Autodesk Inventor part; units mm, degrees
ref_plane "YZ Plane" through (0, 0, 0) normal (1, 0, 0) x (0, 1, 0)
ref_plane "XZ Plane" through (0, 0, 0) normal (0, 1, 0) x (-1, 0, 0)
ref_plane "XY Plane" through (0, 0, 0) normal (0, 0, 1) x (1, 0, 0)
sketch "Sketch1" plane through (0, 0, 0) normal (0, 1, 0) x (-1, 0, 0)
  line L0 (0, 0) -> (-177.8, 0)
  line L1 (-177.8, 0) -> (-177.8, 254)
  line L2 (-177.8, 254) -> (0, 254)
  line L3 (0, 254) -> (0, 0)
  dimension "d0" = 177.8
  dimension "d1" = 254
extrude "Extrusion1" add sketch "Sketch1" along normal blind 127
shell "Shell1" thickness 3.81 removed faces 1 at (118.5333, 127, 169.3333)
sketch "Sketch2" plane through (0, 0, 254) normal (0, 0, 1) x (1, 0, 0)
  line L0 (0, 0) -> (177.8, 0)
  line L1 (177.8, 0) -> (177.8, 127)
  line L2 (0, 127) -> (177.8, 127)
  line L3 (0, 0) -> (0, 127)
extrude "Extrusion2" cut sketch "Sketch2" against normal up to surface (3.81 mm away)
sketch "Sketch3" plane through (0, 0, 0) normal (0, -1, 0) x (1, 0, 0)
  line L0 (177.8, 250.19) -> (0, 250.19)
  line L1 (0, 0) -> (0, 250.19)
  line L2 (177.8, 0) -> (0, 0)
  line L3 (177.8, 250.19) -> (177.8, 0)
  line L4 (177.8, 250.19) -> (0, 250.19)
  line L5 (0, 0) -> (0, 250.19)
  line L6 (177.8, 0) -> (0, 0)
  line L7 (177.8, 250.19) -> (177.8, 0)
  line L8 (177.8, 250.19) -> (177.8, 0)
  spline S0 degree 4 poles (88.9, 250.19) (64.6184, 235.605) (118.3851, 244.1086) (81.3712, 187.8473) (79.1664, 164.6282) (100.7722, 157.4816) (94.5532, 141.1288) (75.1172, 136.7588) (92.4319, 127.4973) (95.6269, 113.3719) (72.1361, 104.6051) (96.8499, 82.5804) (92.3371, 68.5262) (76.0031, 58.8905) (95.1922, 46.8111) (88.2393, 30.5759) (70.5928, 15.1042) (112.5447, 15.7388) (88.9, 0) knots 0 0 0 0 0 0.160311 0.22783 0.291752 0.343709 0.393485 0.441731 0.491587 0.546869 0.603873 0.660906 0.71719 0.768135 0.818353 0.868814 1 1 1 1 1
  spline S1 degree 4 poles (0, 125.095) (-6.7527, 130.6116) (46.7852, 140.872) (29.9087, 101.3612) (79.7395, 129.7272) (116.5747, 129.6492) (130.5567, 112.1302) (157.3819, 135.4422) (165.3765, 119.4615) (177.8, 125.095) knots 0 0 0 0 0 0.260408 0.392164 0.513635 0.63886 0.751218 1 1 1 1 1
  point P0 (83.696, 239.0199)
  point P1 (95.7292, 222.4771)
  point P2 (82.8296, 179.2151)
  point P3 (85.8648, 164.5428)
  point P4 (95.9821, 154.1745)
  point P5 (91.1764, 142.7929)
  point P6 (82.3237, 135.7143)
  point P7 (88.9, 127.3714)
  point P8 (91.4293, 116.2479)
  point P9 (82.0708, 103.6056)
  point P10 (91.9352, 81.8518)
  point P11 (88.9, 68.1851)
  point P12 (83.0825, 58.3094)
  point P13 (90.6705, 46.414)
  point P14 (88.9, 35.0509)
  point P15 (83.696, 23.6656)
  point P16 (92.3673, 15.4774)
  point P17 (7.7387, 130.6712)
  point P18 (36.1302, 125.095)
  point P19 (45.4777, 117.014)
  point P20 (78.8552, 125.095)
  point P21 (117.0831, 125.095)
  point P22 (130.5534, 121.195)
  point P23 (147.0022, 125.095)
  point P24 (161.5605, 125.095)
  point P25 (177.8, 125.095)
  point P26 (88.946, 127.3179)
  point P27 (88.9, 250.19)
  point P28 (88.9, 0)
  point P29 (0, 127.787)
properties part number "Component box Bottom tall"
Verification items for the finished model (mm, model axes). A direction names the side the tool comes from. Coordinates: 2 decimals unless noted, no trailing zeros. Order: outer loops, then holes, each group sorted by start corner. A loop starts at its lowest first (then second) coordinate and runs counter-clockwise, first axis right, second up.
Item 1: Release check for a two-part mould opening along X. For faces 3 (the face through (88, 3, 250.19)), 4 (the face through (173.99, 65, 125)), 5 (the face through (90, 3.81, 129)), 6 (the face through (177.8, 63, 123)) record: +X half, -X half, draft (parallel to the pull), parting line (faces both ways), or undercut.
Filled in:
face 3: draft
face 4: undercut
face 5: undercut
face 6: +X half
Item 2: Access from +Z, -Z, +X, -X, +Y, -Y to the whole of each face (thin tool, end or side, straight path). Record for faces 1 (the face through (3.81, 65, 129)), 2 (the face through (0, 63, 127)).
Filled in:
face 1: +Z, +Y
face 2: +Z, -Z, -X, +Y, -Y
Item 3: Section check C-C, the plane x = 18. Enter the section's corners in (y, z).
Filled in:
outline: (0, 0) - (127, 0) - (127, 3.81) - (3.81, 3.81) - (3.81, 250.19) - (0, 250.19) - close
Item 4: Depth check by flat-ended pin: pin 1 (5 mm diameter, centred on x = 45.5, z = 152.5, fed in from +Y); pin 2 (2 mm diameter, centred on x = 65, y = 24, fed in from +Z). Enter the tip coordinate at first touch or a pass-through.
Filled in:
pin 1: stops at y = 3.81
pin 2: stops at z = 3.81
Item 5: Section check A-A, the plane y = 31. Enter the section's corners in (x, z), then the cut area to 3 significant figures.
Filled in:
outline: (0, 0) - (177.8, 0) - (177.8, 250.19) - (173.99, 250.19) - (173.99, 3.81) - (3.81, 3.81) - (3.81, 250.19) - (0, 250.19) - close
area: 2,550 mm2
Item 6: Material ranges on L1, parallel to X at y = 87.5, z = 110; L2, parallel to Z at x = 35.5, y = 114.5, recorded low to high.
Filled in:
L1: x = 0 to 3.81, 173.99 to 177.8
L2: z = 0 to 3.81
Item 7: Section check B-B, the plane z = 65.5. Enter the section's corners in (x, y), then the cut area to 3 significant figures.
Filled in:
outline: (0, 0) - (177.8, 0) - (177.8, 127) - (173.99, 127) - (173.99, 3.81) - (3.81, 3.81) - (3.81, 127) - (0, 127) - close
area: 1,620 mm2
